from build123d import *

# Parameters (mm, degrees)
SKETCH2_W           = 200
SKETCH2_H           = 80
BOSS_EXTRUDE3_DEPTH = 37
SHELL2_T            = -2
SKETCH3_W           = 122
SKETCH3_H           = 59.69
CUT_EXTRUDE1_DEPTH  = 2
SKETCH4_W           = 200
SKETCH4_H           = 80
BOSS_EXTRUDE4_DEPTH = 2
FILLET5_R           = 2
SKETCH7_W           = 6.575531056
SKETCH7_H           = 5
CUT_EXTRUDE2_DEPTH  = 5
FILLET6_R           = 2


with BuildPart() as part:
    # Sketch2 → Boss-Extrude3 (new body)
    with BuildSketch(Plane(origin=(0, 0, 0), x_dir=(1, 0, 0), z_dir=(0, 1, 0))):
        Rectangle(SKETCH2_W, SKETCH2_H)
    extrude(amount=BOSS_EXTRUDE3_DEPTH)

    # Shell2
    shell2_openings = [part.faces().sort_by_distance(p)[0] for p in [
        (0, 37, 0),
    ]]
    offset(amount=SHELL2_T, openings=shell2_openings, kind=Kind.INTERSECTION)

    # Sketch3 → Cut-Extrude1 (cut)
    with BuildSketch(Plane(origin=(0, 2, 0), x_dir=(1, 0, 0), z_dir=(0, 1, 0))):
        Rectangle(SKETCH3_W, SKETCH3_H)
    extrude(amount=-CUT_EXTRUDE1_DEPTH, mode=Mode.SUBTRACT)

    # Sketch4 → Boss-Extrude4 (add)
    with BuildSketch(Plane.XZ):
        Rectangle(SKETCH4_W, SKETCH4_H)
    extrude(amount=BOSS_EXTRUDE4_DEPTH)

    # Fillet5
    fillet5_edges = [part.edges().sort_by_distance(p)[0] for p in [
        (-61, 1, 29.845),
        (-61, 1, -29.845),
        (61, 1, -29.845),
        (61, 1, 29.845),
    ]]
    fillet(fillet5_edges, radius=FILLET5_R)

    # Sketch7 → Cut-Extrude2 (cut)
    with BuildSketch(Plane.ZY.offset(100)):
        with Locations((23.042234472, 34.5)):
            Rectangle(SKETCH7_W, SKETCH7_H)
    extrude(amount=-CUT_EXTRUDE2_DEPTH, mode=Mode.SUBTRACT)

    # Fillet6
    fillet6_edges = [part.edges().sort_by_distance(p)[0] for p in [
        (-100, 34.5, 26.33),
        (-100, 34.5, 19.754468944),
        (-100, 32, 23.042234472),
    ]]
    fillet(fillet6_edges, radius=FILLET6_R - 0.0001)  # a hair under: the kernel refuses the full size


solid = part.part
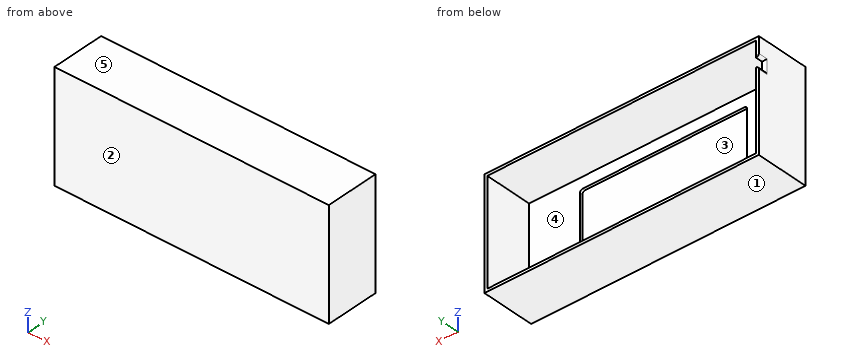
The listing builds one solid part. Answer for the finished solid, in the listing's coordinates (mm). Face numbers are marked on the shaded views. A direction names the side the tool comes from. Coordinates: 2 decimals unless noted, no trailing zeros. Order: outer loops, then holes, each group sorted by start corner. A loop starts at its lowest first (then second) coordinate and runs counter-clockwise, first axis right, second up.
Q1. A cutting plane is placed at C-C, the plane z = -33. Write down the section's boundary in (x, y).
Q2. Given P1, Ø1, axis at x = 29.5, z = 4.5, coming from the +Y side, flat-ended and moving along its own axis, determine where the tip first touches the part or whether it passes through.
Q3. A cutting plane is placed at D-D, the plane x = -5.5. Write down the section's boundary in (y, z) (3 decimals), and give its area (3 significant figures).
Q4. Which of the six approach directions +Z, -Z, +X, -X, +Y, -Y give full straight-line access (tool end or side, diameter ignored) to the marked faces 4 and 5?
Q5. Consider line 1 (X direction, y = 20, z = -27.5); line 2 (X direction, y = 0.5, z = 14); line 3 (Z direction, x = -79, y = 8). Determine where each line is inside the solid, lowest interval first.
Q6. A cutting plane is placed at A-A, the plane y = 16.5. Write down the section's boundary in (x, z).
Q7. For a pull along Z with two mould halves and no side action, classify the marked faces 1, 2 and 3 as pulls with the +Z half, pulls with the -Z half, needs draft (parallel to the pull), parting line crosses it, or undercut.
Q8. A cutting plane is placed at B-B, the plane x = -86. Write down the section's boundary in (y, z).
Answers follow:
1. outline: (-100, -2) - (100, -2) - (100, 37) - (98, 37) - (98, 2) - (-98, 2) - (-98, 37) - (-100, 37) - close
2. P1: stops at y = 0
3. outline: (-2, -40) - (37, -40) - (37, -38) - (2, -38) - (2, -29.845) - (0, -29.845) - (0, 29.845) - (2, 29.845) - (2, 38) - (37, 38) - (37, 40) - (-2, 40) - close
3. area: 341 mm2
4. face 4: +Y
4. face 5: +Z, +X, -X, +Y, -Y
5. line 1: x = -100 to -98, 98 to 100
5. line 2: x = -100 to -61, 61 to 100
5. line 3: z = -40 to -38, 38 to 40
6. outline: (-100, -40) - (100, -40) - (100, 40) - (-100, 40) - close; hole (-98, -38) - (98, -38) - (98, 38) - (-98, 38) - close
7. face 1: pulls with the -Z half
7. face 2: needs draft
7. face 3: undercut
8. outline: (-2, -40) - (37, -40) - (37, -38) - (2, -38) - (2, 38) - (37, 38) - (37, 40) - (-2, 40) - close
